```python
from build123d import *

# Parameters (mm, degrees)
SKETCH1_R           = 5
BOSS_EXTRUDE1_DEPTH = 6
SKETCH2_R           = 4
BOSS_EXTRUDE2_DEPTH = 96
SKETCH6_OUTSIDE_W   = 32.596
SKETCH6_OUTSIDE_H   = 32.596
SKETCH6_OUTSIDE_W_2 = 5
SKETCH6_OUTSIDE_H_2 = 16.430986644
CUT_EXTRUDE1_DEPTH  = 96


with BuildPart() as part:
    # Sketch1 → Boss-Extrude1 (new body)
    with BuildSketch(Plane.XY):
        Circle(SKETCH1_R)
    extrude(amount=BOSS_EXTRUDE1_DEPTH)

    # Sketch2 → Boss-Extrude2 (add)
    with BuildSketch(Plane.XY.offset(6)):
        Circle(SKETCH2_R)
    extrude(amount=BOSS_EXTRUDE2_DEPTH)

    # Sketch6 outside → Cut-Extrude1 (cut)
    with BuildSketch(Plane.XY.offset(102)):
        Rectangle(SKETCH6_OUTSIDE_W, SKETCH6_OUTSIDE_H)
        Rectangle(SKETCH6_OUTSIDE_W_2, SKETCH6_OUTSIDE_H_2, mode=Mode.SUBTRACT)
    extrude(amount=-CUT_EXTRUDE1_DEPTH, mode=Mode.SUBTRACT)


solid = part.part
```
Work out the finished part from the listing and answer in its coordinate system (mm). A direction names the side the tool comes from. Give positions to 0.01 mm unless a question says otherwise; leave off trailing zeros. Write each loop counter-clockwise with the first axis right and the second up, starting at its lowest first coordinate (ties: lowest second). Pieces come first, ordered by that corner, then holes. Notation, with made-up numbers: (-37.75, 62.5) -> (19.25, 62.5) arc R26 ccw to (19.25, 82.5) -> close; hole circle Ø3 at (11.5, -28). An arc over 180 degrees is marked (long way). Write each question's results on one line, items separated by ' | '.
1. Each of these flat-tipped pins is pushed along its axis until it touches: pin 1 Ø5 at (y, z) = (-0.5, 30) entering from -X; pin 2 Ø1.9 at (y, z) = (-0.5, 62) entering from +X. Where does it stop, or does it pass through?
Data:
pin 1: x = -2.5 | pin 2: x = 2.5
2. A tool of negligible diameter and unlimited length cuts with its end or side. For faces 1 (the flat face through (-2.5, 0, 55)), 2 (the flat face through (2.5, 0, 55)), 3 (the flat face through (3, 0, 6)), from which of +Z, -Z, +X, -X, +Y, -Y can it reach the whole face along a straight path? Write none if from no direction.
Data:
face 1: +Z, -X, +Y, -Y | face 2: +Z, +X, +Y, -Y | face 3: +Z
3. Find section B-B on y = 0. Determine the outline of the cut face in (x, z), and give its area (3 significant figures).
Data:
outline: (-5, 0) -> (5, 0) -> (5, 6) -> (2.5, 6) -> (2.5, 102) -> (-2.5, 102) -> (-2.5, 6) -> (-5, 6) -> close | area: 540 mm^2
4. Find section A-A on x = 0. Determine the outline of the cut face in (y, z).
Data:
outline: (-5, 0) -> (5, 0) -> (5, 6) -> (4, 6) -> (4, 102) -> (-4, 102) -> (-4, 6) -> (-5, 6) -> close
5. Straight lines are drawn through the part: L1, parallel to X at y = 2.75, z = 38; L2, parallel to Z at x = -4, y = -0.25; L3, parallel to Y at x = 0, z = 60. For each, find the intervals that lie inside material, in ascending order.
Data:
L1: -2.5 to 2.5 | L2: 0 to 6 | L3: -4 to 4
6. Find section C-C on z = 45.5. Determine the outline of the cut face in (x, y).
Data:
outline: (-2.5, -3.12) arc R4 ccw to (2.5, -3.12) -> (2.5, 3.12) arc R4 ccw to (-2.5, 3.12) -> close
